For this review, take the finished solid that the model builds, in its own axes (mm). Round coordinates to 2 decimals unless told otherwise and drop trailing zeros. Loops run counter-clockwise (first coordinate to the right, second up) from the corner with the lowest first, then second, coordinate; pieces in that order, holes last. Notation, with made-up numbers: (15.25, 21) -> (71.25, 21) arc R22 ccw to (71.25, 54) -> close; hole circle Ø4 at (62, 77). An arc over 180 degrees is marked (long way). Write each question's results on one line, items separated by ' | '.
```python
from build123d import *

# Parameters (mm, degrees)
SKETCH1_W                 = 516.930563546
SKETCH1_H                 = 152.4
BOSS_EXTRUDE1_DEPTH       = 6.35
SKETCH2_W                 = 21.085226308
SKETCH2_H                 = 6.35
SKETCH2_W_2               = 19.05
CUT_EXTRUDE1_DEPTH        = 7.35
LPATTERN1_COUNT           = 3
LPATTERN1_PITCH           = 109.985226308
LPATTERN1_COL_COUNT       = 3
LPATTERN1_COL_PITCH       = 109.985226308
MIRROR1_COPY_1_SKETCH_W   = 21.085226308
MIRROR1_COPY_1_SKETCH_H   = 6.35
MIRROR1_COPY_1_SKETCH_W_2 = 19.05
MIRROR1_COPY_1_DEPTH      = 7.35
MIRROR1_COPY_2_SKETCH_W   = 21.085226308
MIRROR1_COPY_2_SKETCH_H   = 6.35
MIRROR1_COPY_2_SKETCH_W_2 = 19.05
MIRROR1_COPY_2_DEPTH      = 7.35
MIRROR1_COPY_3_SKETCH_W   = 21.085226308
MIRROR1_COPY_3_SKETCH_H   = 6.35
MIRROR1_COPY_3_SKETCH_W_2 = 19.05
MIRROR1_COPY_3_DEPTH      = 7.35
MIRROR1_COPY_4_SKETCH_W   = 21.085226308
MIRROR1_COPY_4_SKETCH_H   = 6.35
MIRROR1_COPY_4_SKETCH_W_2 = 19.05
MIRROR1_COPY_4_DEPTH      = 7.35
CUT_EXTRUDE2_DEPTH        = 7.35


with BuildPart() as part:
    # Sketch1 → Boss-Extrude1 (new body)
    with BuildSketch(Plane(origin=(0, 0, 0), x_dir=(1, 0, 0), z_dir=(0, 1, 0))):
        Rectangle(SKETCH1_W, SKETCH1_H)
    extrude(amount=BOSS_EXTRUDE1_DEPTH)

    # Sketch2 → Cut-Extrude1 (cut, through all)
    with BuildSketch(Plane(origin=(0, 6.35, 0), x_dir=(1, 0, 0), z_dir=(0, 1, 0))):
        with Locations((0, -73.025)):
            Rectangle(SKETCH2_W, SKETCH2_H)
        with Locations((-45.467613154, -73.025)):
            Rectangle(SKETCH2_W_2, SKETCH2_H)
        with Locations((45.467613154, -73.025)):
            Rectangle(SKETCH2_W_2, SKETCH2_H)
    cut_extrude1 = extrude(amount=-CUT_EXTRUDE1_DEPTH, mode=Mode.SUBTRACT)

    # LPattern1: Cut-Extrude1 ×3
    with Locations(*[(i * LPATTERN1_PITCH, 0, 0) for i in range(1, LPATTERN1_COUNT)]):
        add(cut_extrude1, mode=Mode.SUBTRACT)

    # LPattern1 col: Cut-Extrude1 ×3
    with Locations(*[(-i * LPATTERN1_COL_PITCH, 0, 0) for i in range(1, LPATTERN1_COL_COUNT)]):
        add(cut_extrude1, mode=Mode.SUBTRACT)

    # Mirror1: Cut-Extrude1 across plane
    add(cut_extrude1.mirror(Plane.XY), mode=Mode.SUBTRACT)

    # Mirror1 copy 1 sketch → Mirror1 copy 1 (cut, through all)
    with BuildSketch(Plane(origin=(109.985226308, 6.35, 0), x_dir=(1, 0, 0), z_dir=(0, 1, 0))):
        with Locations((0, 73.025)):
            Rectangle(MIRROR1_COPY_1_SKETCH_W, MIRROR1_COPY_1_SKETCH_H)
        with Locations((-45.467613154, 73.025)):
            Rectangle(MIRROR1_COPY_1_SKETCH_W_2, MIRROR1_COPY_1_SKETCH_H)
        with Locations((45.467613154, 73.025)):
            Rectangle(MIRROR1_COPY_1_SKETCH_W_2, MIRROR1_COPY_1_SKETCH_H)
    extrude(amount=-MIRROR1_COPY_1_DEPTH, mode=Mode.SUBTRACT)

    # Mirror1 copy 2 sketch → Mirror1 copy 2 (cut, through all)
    with BuildSketch(Plane(origin=(219.970452616, 6.35, 0), x_dir=(1, 0, 0), z_dir=(0, 1, 0))):
        with Locations((0, 73.025)):
            Rectangle(MIRROR1_COPY_2_SKETCH_W, MIRROR1_COPY_2_SKETCH_H)
        with Locations((-45.467613154, 73.025)):
            Rectangle(MIRROR1_COPY_2_SKETCH_W_2, MIRROR1_COPY_2_SKETCH_H)
        with Locations((45.467613154, 73.025)):
            Rectangle(MIRROR1_COPY_2_SKETCH_W_2, MIRROR1_COPY_2_SKETCH_H)
    extrude(amount=-MIRROR1_COPY_2_DEPTH, mode=Mode.SUBTRACT)

    # Mirror1 copy 3 sketch → Mirror1 copy 3 (cut, through all)
    with BuildSketch(Plane(origin=(-109.985226308, 6.35, 0), x_dir=(1, 0, 0), z_dir=(0, 1, 0))):
        with Locations((0, 73.025)):
            Rectangle(MIRROR1_COPY_3_SKETCH_W, MIRROR1_COPY_3_SKETCH_H)
        with Locations((-45.467613154, 73.025)):
            Rectangle(MIRROR1_COPY_3_SKETCH_W_2, MIRROR1_COPY_3_SKETCH_H)
        with Locations((45.467613154, 73.025)):
            Rectangle(MIRROR1_COPY_3_SKETCH_W_2, MIRROR1_COPY_3_SKETCH_H)
    extrude(amount=-MIRROR1_COPY_3_DEPTH, mode=Mode.SUBTRACT)

    # Mirror1 copy 4 sketch → Mirror1 copy 4 (cut, through all)
    with BuildSketch(Plane(origin=(-219.970452616, 6.35, 0), x_dir=(1, 0, 0), z_dir=(0, 1, 0))):
        with Locations((0, 73.025)):
            Rectangle(MIRROR1_COPY_4_SKETCH_W, MIRROR1_COPY_4_SKETCH_H)
        with Locations((-45.467613154, 73.025)):
            Rectangle(MIRROR1_COPY_4_SKETCH_W_2, MIRROR1_COPY_4_SKETCH_H)
        with Locations((45.467613154, 73.025)):
            Rectangle(MIRROR1_COPY_4_SKETCH_W_2, MIRROR1_COPY_4_SKETCH_H)
    extrude(amount=-MIRROR1_COPY_4_DEPTH, mode=Mode.SUBTRACT)

    # Sketch3 → Cut-Extrude2 (cut, through all)
    with BuildSketch(Plane(origin=(0, 6.35, 0), x_dir=(1, 0, 0), z_dir=(0, 1, 0))):
        Polygon((219.970452616, 69.85), (219.970452616, -76.2), (258.465281773, -76.2), (258.465281773, 76.2), (219.970452616, 76.2), align=None)
    extrude(amount=-CUT_EXTRUDE2_DEPTH, mode=Mode.SUBTRACT)


solid = part.part
```
1. For pin 1 (1.9 mm diameter, centred on x = -106, y = 2.5, fed in from -Z); pin 2 (3 mm diameter, centred on y = 3, z = -74, fed in from -X); pin 3 (1.9 mm diameter, centred on y = 4.5, z = 74, fed in from +X), all flat-tipped, find the tip position at first contact; note any pin that passes through.
Values found:
pin 1: stops at z = -69.85 | pin 2: stops at x = -255.91 | pin 3: stops at x = 209.43
2. Consider section A-A (x = 172.5). State the section outline as (y, z) points.
Values found:
outline: (0, -69.85) -> (6.35, -69.85) -> (6.35, 69.85) -> (0, 69.85) -> close
3. To check wall thickness, follow probe 1 along Z at (x, y) = (-3, 2.5). State the ranges of the line that lie inside material, in increasing order.
Values found:
probe 1: z = -69.85 to 69.85
